Build history of the part. All positions in model axes, mm. A direction names the side the tool comes from. Round coordinates to 2 decimals unless told otherwise and drop trailing zeros. Write each loop counter-clockwise with the first axis right and the second up, starting at its lowest first coordinate (ties: lowest second). Pieces come first, ordered by that corner, then holes.
1) Saw through at D-D (x = 13). Write the cut outline in (y, z).
2) Wall check: probe 1 along Y at (x, z) = (31.5, 12.7); probe 2 along Y at (x, z) = (13.5, 12.5); probe 3 along X at (y, z) = (11, 7.75). Give the ranges that are in metal, low to high.
3) Flat gauge pins, fed straight in: pin 1 (4.5 mm diameter, centred on y = 7, z = 12, fed in from +X); pin 2 (8.5 mm diameter, centred on x = -4.5, z = 14.5, fed in from -Y); pin 3 (3.5 mm diameter, centred on y = 4.572, z = 12.7, fed in from +X); pin 4 (8 mm diameter, centred on y = 8, z = 20, fed in from -X). Where does each tip first touch, or does it go through?
4) Saw through at A-A (z = 12.7). Write the cut outline in (x, y), plus the area to 3 significant figures.
5) Saw through at C-C (x = -1). Write the cut outline in (y, z), plus the area to 3 significant figures.
6) Which spindle directions (+Z, -Z, +X, -X, +Y, -Y) get a long thin tool onto all of the face, cutting with end or side? Do faces 5 (the flat face through (-4, 12.7, 13)), 6 (the flat face through (39, 12.7, 13)), 7 (the cylindrical face through (-3.863, 13.464, 0.724)), 8 (the cylindrical face through (39.317, 13.464, 24.676)), 9 (the cylindrical face through (39.317, 13.464, 0.724)). Say none if no direction does.
7) Saw through at B-B (y = 2). Write the cut outline in (x, z), plus the area to 3 significant figures.
8) Pull direction X, two halves, no side cores. Call faces 1 (the flat face through (21.59, 8, 13)), 2 (the flat face through (13.97, 8, 13)), 3 (the flat face through (35.56, 8, 13)), 4 (the cylindrical face through (6.887, 0.724, 24.636)): +X half, -X half, draft (parallel to the pull), parting line (faces both ways), or undercut.
from build123d import *

# Parameters (mm, degrees)
BOSS_EXTRUDE1_DEPTH = 25.4
FILLET1_R           = 2.54
SKETCH2_R           = 2.032
CUT_EXTRUDE1_DEPTH  = 54.596407529
FILLET2_R           = 2.54


with BuildPart() as part:
    # Sketch1 → Boss-Extrude1 (new body)
    with BuildSketch(Plane.XY):
        Polygon((0, 0), (0, 12.7), (-7.62, 12.7), (-7.62, 19.05), (43.18, 19.05), (43.18, 12.7), (35.56, 12.7), (35.56, 0), (21.59, 0), (21.59, 12.7), (13.97, 12.7), (13.97, 0), align=None)
    extrude(amount=BOSS_EXTRUDE1_DEPTH)

    # Fillet1
    fillet1_edges = [part.edges().sort_by_distance(p)[0] for p in [
        (28.575, 0, 0),
        (6.985, 0, 0),
        (28.575, 0, 25.4),
        (6.985, 0, 25.4),
    ]]
    fillet(fillet1_edges, radius=FILLET1_R)

    # Sketch2 → Cut-Extrude1 (cut, through all)
    with BuildSketch(Plane(origin=(35.56, 0, 0), x_dir=(0, 0, -1), z_dir=(1, 0, 0))):
        with Locations((-12.7, 4.572)):
            Circle(SKETCH2_R)
    extrude(amount=-CUT_EXTRUDE1_DEPTH, mode=Mode.SUBTRACT)

    # Fillet2
    fillet2_edges = [part.edges().sort_by_distance(p)[0] for p in [
        (17.78, 12.7, 25.4),
        (-3.81, 12.7, 0),
        (39.37, 12.7, 0),
        (17.78, 12.7, 0),
        (39.37, 12.7, 25.4),
        (-3.81, 12.7, 25.4),
    ]]
    fillet(fillet2_edges, radius=FILLET2_R)


solid = part.part
Evaluation:
1. outline: (0, 2.54) arc R2.54 ccw to (2.54, 0) - (19.05, 0) - (19.05, 25.4) - (2.54, 25.4) arc R2.54 ccw to (0, 22.86) - close; hole circle Ø4.06 at (4.57, 12.7)
2. probe 1: y = 0 to 2.54, 6.6 to 19.05
2. probe 2: y = 0 to 2.55, 6.59 to 19.05
2. probe 3: x = 0 to 13.97, 21.59 to 35.56
3. pin 1: stops at x = 35.56
3. pin 2: stops at y = 12.7
3. pin 3: passes through
3. pin 4: stops at x = 0
4. outline: (-7.62, 12.7) - (0, 12.7) - (0, 6.6) - (13.97, 6.6) - (13.97, 12.7) - (21.59, 12.7) - (21.59, 6.6) - (35.56, 6.6) - (35.56, 12.7) - (43.18, 12.7) - (43.18, 19.05) - (-7.62, 19.05) - close; (0, 0) - (13.97, 0) - (13.97, 2.54) - (0, 2.54) - close; (21.59, 0) - (35.56, 0) - (35.56, 2.54) - (21.59, 2.54) - close
4. area: 564 mm2
5. outline: (12.7, 2.54) arc R2.54 ccw to (15.24, 0) - (19.05, 0) - (19.05, 25.4) - (15.24, 25.4) arc R2.54 ccw to (12.7, 22.86) - close
5. area: 159 mm2
6. face 5: +Z, -Z, -X, -Y
6. face 6: +Z, -Z, +X, -Y
6. face 7: -Z, -X, -Y
6. face 8: +Z, +X, -Y
6. face 9: -Z, +X, -Y
7. outline: (0, 0.06) - (13.97, 0.06) - (13.97, 25.34) - (0, 25.34) - close; (21.59, 0.06) - (35.56, 0.06) - (35.56, 25.34) - (21.59, 25.34) - close
7. area: 706 mm2
8. face 1: undercut
8. face 2: undercut
8. face 3: +X half
8. face 4: draft
